from build123d import *

# Parameters (mm, degrees)
SKETCH_1_R      = 10
EXTRUDE_1_DEPTH = 16.4
SKETCH_2_R      = 0.8
EXTRUDE_2_DEPTH = 4.3


with BuildPart() as part:
    # Эскиз1 → Бобышка-Вытянуть1 (new body)
    with BuildSketch(Plane(origin=(0, 0, 0), x_dir=(1, 0, 0), z_dir=(0, 1, 0))):
        with Locations(Location((0, 0, 0), (0, 0, 270))):
            Circle(SKETCH_1_R)
    extrude(amount=EXTRUDE_1_DEPTH)

    # Эскиз2 → Бобышка-Вытянуть2 (add)
    with BuildSketch(Plane.XZ):
        with Locations(Location((0, 6.75, 0), (0, 0, 90))):
            Circle(SKETCH_2_R)
        with Locations(Location((-6.75, 0, 0), (0, 0, 90))):
            Circle(SKETCH_2_R)
    extrude(amount=EXTRUDE_2_DEPTH)


solid = part.part
Read the model definition and answer for the solid it produces. Units are mm, in the model's axes. A direction names the side the tool comes from. Give positions to 0.01 mm unless a question says otherwise; leave off trailing zeros. Write each loop counter-clockwise with the first axis right and the second up, starting at its lowest first coordinate (ties: lowest second). Pieces come first, ordered by that corner, then holes. Notation, with made-up numbers: M 15.5,-18 L 68.5,-18 A14 ccw 68.5,-5 Z; hole C 37.25,18 d10. An arc over 180 degrees is marked long. One line per item, written item: value. Start each with the question number.
(1) Find section B-B (x = 0). Determine the outline of the cut face in (y, z), plus the area to 3 significant figures.
(2) Flat-ended cylindrical pins translate along their axes: pin 1 Ø8 at (x, y) = (8, 6) entering from +Z; pin 2 Ø1 at (x, y) = (4, 6.5) entering from -Z; pin 3 Ø8 at (x, y) = (7, 7) entering from +Z. Find the tip coordinate at first contact, or state that the pin passes through.
(3) Find the intervals of material crossed by line 1 (Y direction, x = 4, z = -8); line 2 (X direction, y = 2.5, z = 0); line 3 (X direction, y = 9, z = 3.5), in increasing order.
(4) Determine the mould class of faces 1 (the cylindrical face through (-7.543, -2.12, -0.104)), 2 (the flat face through (0, 0, 0)), 3 (the flat face through (0, 16.4, 0)) for opening direction Y: pulls with the +Y half, pulls with the -Y half, needs draft (parallel to the pull), parting line crosses it, or undercut.
(5) Find section C-C (y = -2.5). Determine the outline of the cut face in (x, z).
(6) Find section A-A (z = 0). Determine the outline of the cut face in (x, y).
(7) A tool of negligible diameter and unlimited length cuts with its end or side. For faces 4 (the flat face through (-7, -4.3, 0)), 5 (the cylindrical face through (-0.04, -2.12, 5.95)), from which of +Z, -Z, +X, -X, +Y, -Y can it reach the whole face along a straight path? Write none if from no direction.
(8) Find section D-D (y = 14.25). Determine the outline of the cut face in (x, z), plus the area to 3 significant figures.
Results below:
1. outline: M -4.3,5.95 L 0,5.95 L 0,-10 L 16.4,-10 L 16.4,10 L 0,10 L 0,7.55 L -4.3,7.55 Z
1. area: 335 mm^2
2. pin 1: stops at z = 9.17
2. pin 2: stops at z = -9.37
2. pin 3: stops at z = 9.54
3. line 1: y = 0 to 16.4
3. line 2: x = -10 to 10
3. line 3: x = -9.37 to 9.37
4. face 1: needs draft
4. face 2: pulls with the -Y half
4. face 3: pulls with the +Y half
5. outline: C -6.75,0 d1.6; C 0,6.75 d1.6
6. outline: M -10,0 L -7.55,0 L -7.55,-4.3 L -5.95,-4.3 L -5.95,0 L 10,0 L 10,16.4 L -10,16.4 Z
7. face 4: +Z, -Z, +X, -X, -Y
7. face 5: -Y
8. outline: C 0,0 d20
8. area: 314 mm^2
